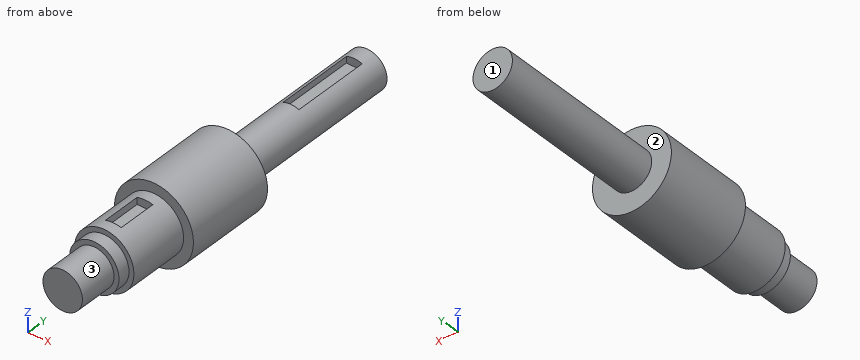
from build123d import *

# Parameters (mm, degrees)
F0_R      = 10
F1_DEPTH  = 88
F2_R      = 20
F3_DEPTH  = 46.825
F4_R      = 15
F5_DEPTH  = 31.4
F6_R      = 12.5
F7_DEPTH  = 6.325
F8_R      = 10
F9_DEPTH  = 20
F11_W     = 4
F11_H     = 40
F11_H_2   = 20
F12_DEPTH = 4
F14_W     = 4
F14_H     = 20
F15_DEPTH = 4


with BuildPart() as f1:
    # F0 (on Front) → F1 (new body)
    with BuildSketch(Plane.XZ):
        Circle(F0_R)
    extrude(amount=F1_DEPTH)

    # F2 (on face) → F3 (join)
    with BuildSketch(Plane.XZ.offset(88)):
        Circle(F2_R)
    extrude(amount=F3_DEPTH)

    # F4 (on face) → F5 (join)
    with BuildSketch(Plane.XZ.offset(134.825)):
        Circle(F4_R)
    extrude(amount=F5_DEPTH)

    # F6 (on face) → F7 (join)
    with BuildSketch(Plane.XZ.offset(166.225)):
        Circle(F6_R)
    extrude(amount=F7_DEPTH)

    # F8 (on face) → F9 (join)
    with BuildSketch(Plane.XZ.offset(172.55)):
        Circle(F8_R)
    extrude(amount=F9_DEPTH)

    # F11 (on offset) → F12 (cut)
    with BuildSketch(Plane.XY.offset(10)):
        with Locations((2, -28.240694)):
            Rectangle(F11_W, F11_H)
        with Locations((-2, -28.240694)):
            Rectangle(F11_W, F11_H)
        with Locations((-2, -150.525)):
            Rectangle(F11_W, F11_H_2)
        with Locations((2, -150.525)):
            Rectangle(F11_W, F11_H_2)
    extrude(amount=-F12_DEPTH, mode=Mode.SUBTRACT)

    # F14 (on offset) → F15 (cut)
    with BuildSketch(Plane.XY.offset(15)):
        with Locations((-2, -150.525)):
            Rectangle(F14_W, F14_H)
        with Locations((2, -150.525)):
            Rectangle(F14_W, F14_H)
    extrude(amount=-F15_DEPTH, mode=Mode.SUBTRACT)


solid = f1.part
The listing builds one solid part. Answer for the finished solid, in the listing's coordinates (mm). Face numbers are marked on the shaded views. A direction names the side the tool comes from. Give positions to 0.01 mm unless a question says otherwise; leave off trailing zeros. Write each loop counter-clockwise with the first axis right and the second up, starting at its lowest first coordinate (ties: lowest second). Pieces come first, ordered by that corner, then holes.
Item 1: Which of the six approach directions +Z, -Z, +X, -X, +Y, -Y give full straight-line access (tool end or side, diameter ignored) to the marked faces 1, 2 and 3?
Item 2: Section B-B, the plane z = 0 is taken. Write down the section's boundary in (x, y) (3 decimals), plus the area to 3 significant figures.
Item 3: Find the intervals of material crossed by line 1 along Y through (x, z) = (-3, 7) (3 decimals); line 2 along Y through (x, z) = (8, 11) (3 decimals); line 3 along Y through (x, z) = (17, -7.5) (3 decimals), in increasing order.
Item 4: Flat-ended cylindrical pins translate along their axes: P1, Ø2, axis at x = -8, y = -150, coming from the +Z side; P2, Ø1.2, axis at x = 0, z = 13.5, coming from the +Y side; P3, Ø2.5, axis at x = 0.5, y = -150, coming from the -Z side. Find the tip coordinate at first contact, or state that the pin passes through.
Item 5: Section C-C, the plane y = -104.5 is taken. Write down the section's boundary in (x, z), plus the area to 3 significant figures.
Completed:
1. face 1: +Z, -Z, +X, -X, +Y
1. face 2: +Y
1. face 3: -Y
2. outline: (-20, -134.825) - (-15, -134.825) - (-15, -166.225) - (-12.5, -166.225) - (-12.5, -172.55) - (-10, -172.55) - (-10, -192.55) - (10, -192.55) - (10, -172.55) - (12.5, -172.55) - (12.5, -166.225) - (15, -166.225) - (15, -134.825) - (20, -134.825) - (20, -88) - (10, -88) - (10, 0) - (-10, 0) - (-10, -88) - (-20, -88) - close
2. area: 5,130 mm2
3. line 1: y = -192.55 to -160.525, -140.525 to -48.241, -8.241 to 0
3. line 2: y = -166.225 to -88
3. line 3: y = -134.825 to -88
4. P1: stops at z = 13.27
4. P2: stops at y = -88
4. P3: stops at z = -15
5. outline: circle Ø40 at (0, 0)
5. area: 1,260 mm2
